Could you check a few things on this drawing? It's one solid part, dimensions in mm from its lowest x, y, z. Give positions to 0.01 mm unless a question says otherwise; leave off trailing zeros. Write each loop counter-clockwise with the first axis right and the second up, starting at its lowest first coordinate (ties: lowest second). Pieces come first, ordered by that corner, then holes.
1. If I drill on probe 1 along Z at (x, y) = (165.5, 0.45); probe 2 along Z at (x, y) = (87, 1.9), over which ranges is the centre line in solid material (lowest first)?
2. I'm going to push a flat-ended pin straight in: pin 1 (12 mm diameter, centred on x = 161.5, z = 104, fed in from -Y). Where does the tip first touch, or does it pass through?
3. Suppose I cut it at B-B (y = 1.95). Please give me the cut outline in (x, z), and give its area (3 significant figures).
4. Suppose I cut it at A-A (x = 105.5). Please give me the cut outline in (y, z).
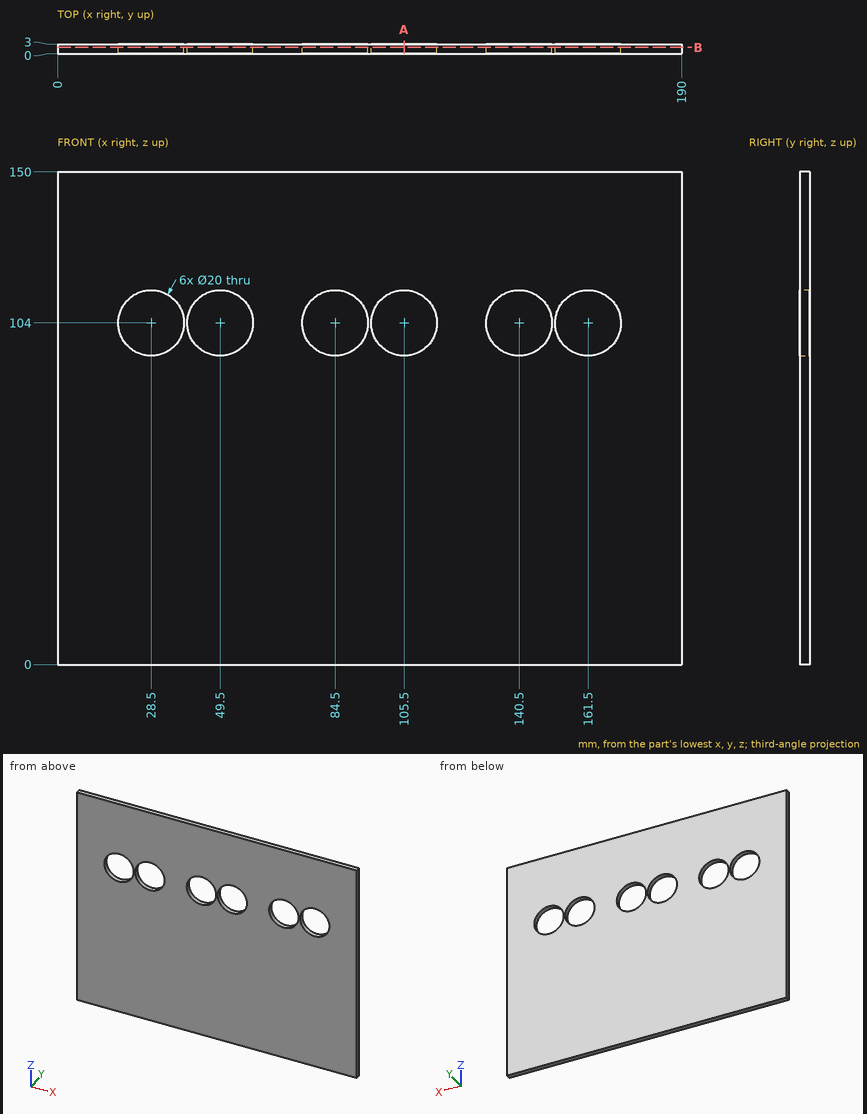
Checks:
1. probe 1: z = 0 to 94.83, 113.17 to 150
1. probe 2: z = 0 to 94.32, 113.68 to 150
2. pin 1: passes through
3. outline: (0, 0) - (190, 0) - (190, 150) - (0, 150) - close; hole circle Ø20 at (28.5, 104); hole circle Ø20 at (49.5, 104); hole circle Ø20 at (84.5, 104); hole circle Ø20 at (105.5, 104); hole circle Ø20 at (140.5, 104); hole circle Ø20 at (161.5, 104)
3. area: 26,600 mm2
4. outline: (0, 0) - (3, 0) - (3, 94) - (0, 94) - close; (0, 114) - (3, 114) - (3, 150) - (0, 150) - close
